from build123d import *

# Parameters (mm, degrees)
BOSS_EXTRUDE2_DEPTH = 20
SKETCH4_W           = 10
SKETCH4_H           = 20
CUT_EXTRUDE1_DEPTH  = 50


with BuildPart() as part:
    # Sketch1 → Boss-Extrude2 (new body)
    with BuildSketch(Plane(origin=(0, 0, 0), x_dir=(1, 0, 0), z_dir=(0, 1, 0))):
        with BuildLine():
            Line((-80.69665409, 52.02034588), (-35.69665409, 52.02034588))
            ThreePointArc((-35.69665409, 52.02034588), (-28.625586278, 54.949278068), (-25.69665409, 62.02034588))
            Line((-25.69665409, 62.02034588), (-25.69665409, 102.02034588))
            Line((-25.69665409, 102.02034588), (15.30334591, 102.02034588))
            Line((15.30334591, 102.02034588), (15.30334591, 62.02034588))
            ThreePointArc((15.30334591, 62.02034588), (18.232278099, 54.949278068), (25.30334591, 52.02034588))
            Line((25.30334591, 52.02034588), (70.30334591, 52.02034588))
            Line((70.30334591, 52.02034588), (70.30334591, 42.02034588))
            Line((70.30334591, 42.02034588), (-80.69665409, 42.02034588))
            Line((-80.69665409, 42.02034588), (-80.69665409, 52.02034588))
        make_face()
    extrude(amount=BOSS_EXTRUDE2_DEPTH)

    # Sketch4 → Cut-Extrude1 (cut)
    with BuildSketch(Plane(origin=(0, 0, -102.02034588), x_dir=(-1, 0, 0), z_dir=(0, 0, -1))):
        with Locations((5.19665409, 10)):
            Rectangle(SKETCH4_W, SKETCH4_H)
    extrude(amount=-CUT_EXTRUDE1_DEPTH, mode=Mode.SUBTRACT)


solid = part.part
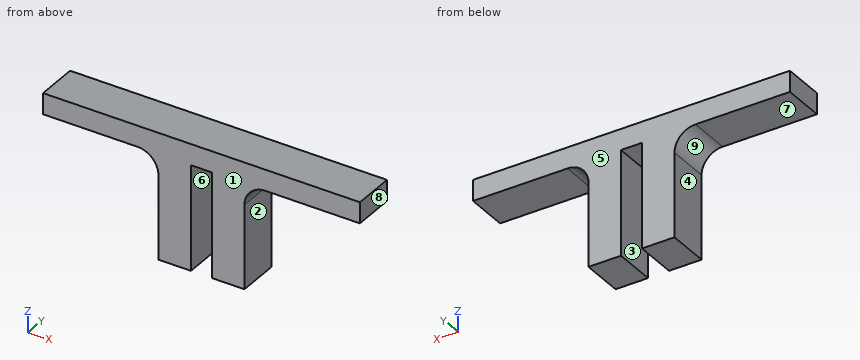
Read the model definition and answer for the solid it produces. Units are mm, in the model's axes. Face numbers are marked on the shaded views. A direction names the side the tool comes from. Give positions to 0.01 mm unless a question says otherwise; leave off trailing zeros. Loops run counter-clockwise (first coordinate to the right, second up) from the corner with the lowest first, then second, coordinate; pieces in that order, holes last. Notation, with made-up numbers: (-31.5, -35.5) -> (-23.5, -35.5) arc R4 cw to (-23.5, -30.5) -> close; hole circle Ø4 at (-24.75, 31.25). An arc over 180 degrees is marked (long way). Answer as CSV lines item,"result".
Item 1: Find section B-B on y = 17.5. Give the vertices of the cut face in (x, z).
Returned:
outline,"(-80.7, -52.02) -> (-35.7, -52.02) arc R10 cw to (-25.7, -62.02) -> (-25.7, -102.02) -> (-10.2, -102.02) -> (-10.2, -52.02) -> (-0.2, -52.02) -> (-0.2, -102.02) -> (15.3, -102.02) -> (15.3, -62.02) arc R10 cw to (25.3, -52.02) -> (70.3, -52.02) -> (70.3, -42.02) -> (-80.7, -42.02) -> close"
Item 2: Each of these flat-tipped pins is pushed along its axis until it touches: pin 1 (10 mm diameter, centred on x = 47, y = 11.5, fed in from -Z); pin 2 (5 mm diameter, centred on y = 7.5, z = -93.5, fed in from +X); pin 3 (8 mm diameter, centred on y = 3, z = -62, fed in from +X). Where does it stop, or does it pass through?
Returned:
pin 1,"stops at z = -52.02"
pin 2,"stops at x = 15.3"
pin 3,"stops at x = 16.15"
Item 3: For the marked faces 1, 2, 3, 4 and 5, determine the directions among +Z, -Z, +X, -X, +Y, -Y from which every point of the face is accessible in a straight line to the end or side of a thin tool.
Returned:
face 1,"+Z, -Z, +X, -X, -Y"
face 2,"-Z, +X, +Y, -Y"
face 3,"-Z, +Y, -Y"
face 4,"-Z, -X, +Y, -Y"
face 5,"+Z, -Z, +X, -X, +Y"
Item 4: Find section A-A on z = -84.5. Give the vertices of the cut face in (x, y), plus the area to 3 significant figures.
Returned:
outline,"(-25.7, 0) -> (-10.2, 0) -> (-10.2, 20) -> (-25.7, 20) -> close; (-0.2, 0) -> (15.3, 0) -> (15.3, 20) -> (-0.2, 20) -> close"
area,"620 mm²"
Item 5: Find section D-D on x = -58.5. Give the vertices of the cut face in (y, z).
Returned:
outline,"(0, -52.02) -> (20, -52.02) -> (20, -42.02) -> (0, -42.02) -> close"
Item 6: Determine the mould class of the marked faces 6, 7, 8 and 9 for opening direction X: +X half, -X half, draft (parallel to the pull), parting line (faces both ways), or undercut.
Returned:
face 6,"undercut"
face 7,"draft"
face 8,"+X half"
face 9,"-X half"
Item 7: Consider line 1 (X direction, y = 10.25, z = -71); line 2 (Z direction, x = -55, y = 17.75); line 3 (X direction, y = 14.5, z = -56). Determine where each line is inside the solid, lowest interval first. Write a range as [from, to].
Returned:
line 1,"x = [-25.7, -10.2], [-0.2, 15.3]"
line 2,"z = [-52.02, -42.02]"
line 3,"x = [-27.71, -10.2], [-0.2, 17.32]"
Item 8: Find section C-C on z = -55. Give the vertices of the cut face in (x, y), plus the area to 3 significant figures.
Returned:
outline,"(-28.58, 0) -> (-10.2, 0) -> (-10.2, 20) -> (-28.58, 20) -> close; (-0.2, 0) -> (18.18, 0) -> (18.18, 20) -> (-0.2, 20) -> close"
area,"735 mm²"
